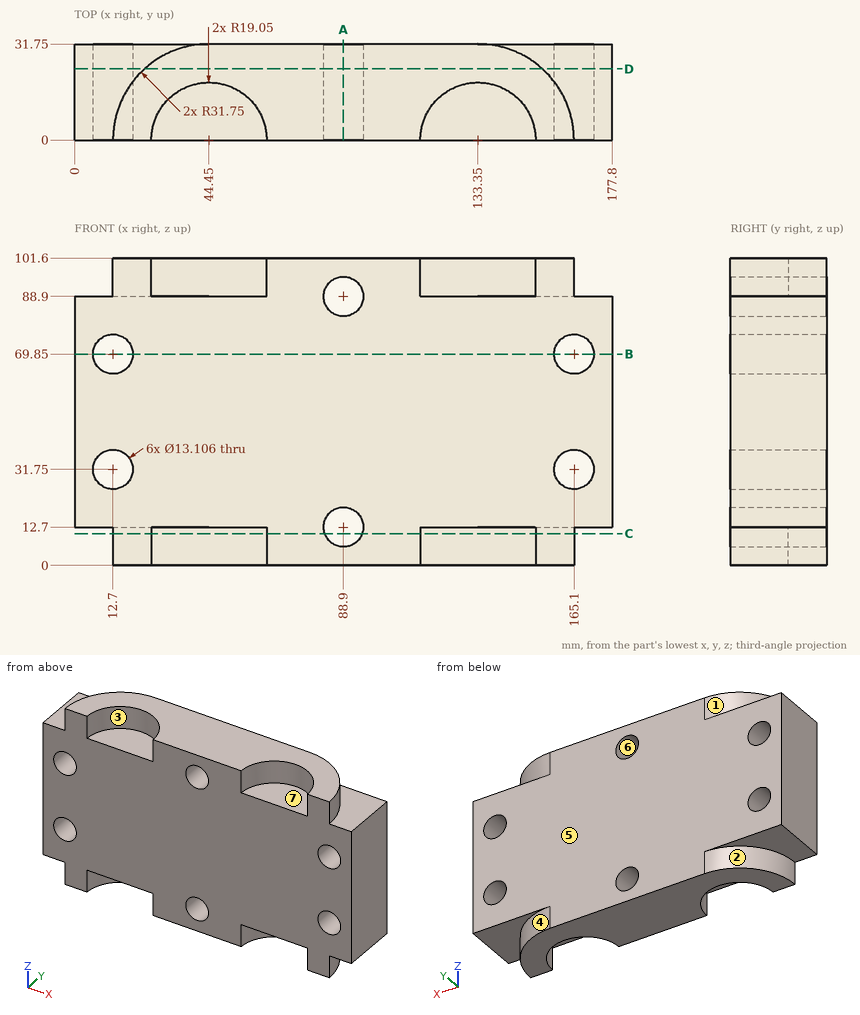
The figure shows three views and two pictorial views of one solid part (mm, origin at its lowest corner). Answer the questions. A direction names the side the tool comes from. Give positions to 0.01 mm unless a question says otherwise; leave off trailing zeros. Write each loop counter-clockwise with the first axis right and the second up, starting at its lowest first coordinate (ties: lowest second). Pieces come first, ordered by that corner, then holes. Notation, with made-up numbers: (32.25, 56.5) -> (51.25, 56.5) arc R16 ccw to (51.25, 77.5) -> close; hole circle Ø11 at (-28.75, 76). An arc over 180 degrees is marked (long way). Use one line per item in the form item = value.
1) Straight lines are drawn through the part: probe 1 along X at (y, z) = (15, 32); probe 2 along Z at (x, y) = (164.5, 28) (1 decimal); probe 3 along Z at (x, y) = (88.9, 10). For each, find the intervals that lie inside material, in ascending order.
Result:
probe_1 = 0 to 6.15, 19.25 to 158.55, 171.65 to 177.8
probe_2 = 12.7 to 25.2, 38.3 to 63.3, 76.4 to 88.9
probe_3 = 0 to 6.15, 19.25 to 82.35, 95.45 to 101.6
2) Section D-D on y = 23.5 is taken. Write down the section's boundary in (x, z).
Result:
outline = (0, 12.7) -> (23.1, 12.7) -> (23.1, 0) -> (154.7, 0) -> (154.7, 12.7) -> (177.8, 12.7) -> (177.8, 88.9) -> (154.7, 88.9) -> (154.7, 101.6) -> (23.1, 101.6) -> (23.1, 88.9) -> (0, 88.9) -> close; hole circle Ø13.11 at (12.7, 31.75); hole circle Ø13.11 at (12.7, 69.85); hole circle Ø13.11 at (88.9, 12.7); hole circle Ø13.11 at (88.9, 88.9); hole circle Ø13.11 at (165.1, 31.75); hole circle Ø13.11 at (165.1, 69.85)
3) Section A-A on x = 88.9 is taken. Write down the section's boundary in (y, z).
Result:
outline = (0, 0) -> (31.75, 0) -> (31.75, 6.15) -> (0, 6.15) -> close; (0, 19.25) -> (31.75, 19.25) -> (31.75, 82.35) -> (0, 82.35) -> close; (0, 95.45) -> (31.75, 95.45) -> (31.75, 101.6) -> (0, 101.6) -> close
4) Section C-C on z = 10.5 is taken. Write down the section's boundary in (x, y).
Result:
outline = (12.7, 0) -> (25.4, 0) arc R19.05 cw to (63.5, 0) -> (82.73, 0) -> (82.73, 31.75) -> (44.45, 31.75) arc R31.75 ccw to start; (95.07, 0) -> (114.3, 0) arc R19.05 cw to (152.4, 0) -> (165.1, 0) arc R31.75 ccw to (133.35, 31.75) -> (95.07, 31.75) -> close
5) Section B-B on z = 69.85 is taken. Write down the section's boundary in (x, y).
Result:
outline = (0, 0) -> (6.15, 0) -> (6.15, 31.75) -> (0, 31.75) -> close; (19.25, 0) -> (158.55, 0) -> (158.55, 31.75) -> (19.25, 31.75) -> close; (171.65, 0) -> (177.8, 0) -> (177.8, 31.75) -> (171.65, 31.75) -> close
6) For a pull along Z with two mould halves and no side action, classify the marked faces 5, 6 and 7 as +Z half, -Z half, draft (parallel to the pull), parting line (faces both ways), or undercut.
Result:
face_5 = draft
face_6 = undercut
face_7 = +Z half
7) Each of these flat-tipped pins is pushed along its axis until it touches: P1, Ø15, axis at x = 48.5, y = 9, coming from the +Z side; P2, Ø1.5, axis at y = 13.5, z = 10.5, coming from the +X side; P3, Ø8, axis at x = 12.7, z = 31.75, coming from the +Y side; P4, Ø9.5, axis at x = 47, y = 12, coming from the -Z side. Where does it stop, or does it pass through?
Result:
P1 = 88.9
P2 = 162.43
P3 = through
P4 = 12.7
8) A tool of negligible diameter and unlimited length cuts with its end or side. For the marked faces 1, 2, 3 and 4, from which of +Z, -Z, +X, -X, +Y, -Y can it reach the whole face along a straight path? Write none if from no direction.
Result:
face_1 = +Z, -X, +Y
face_2 = -Z, -X, +Y
face_3 = +Z, -Y
face_4 = -Z, +X, +Y
